Design review of the part built by this model. Coordinates are the model's own, in mm. A direction names the side the tool comes from. Coordinates: 2 decimals unless noted, no trailing zeros. Loops run counter-clockwise (first coordinate to the right, second up) from the corner with the lowest first, then second, coordinate; pieces in that order, holes last. Notation, with made-up numbers: (-7, 41.25) -> (8, 41.25) arc R5 cw to (8, 49.25) -> close; hole circle Ø9 at (73, 1). An arc over 180 degrees is marked (long way). One line per item, written item: value. Start each with the question number.
1. For probe 1 along Y at (x, z) = (9.5, 1); probe 2 along Y at (x, z) = (8, 16); probe 3 along Y at (x, z) = (9.75, 11), list the stretches that pass through material, from the lowest coordinate up.
2. Add section A-A on y = 52. Write out the cut boundary in (x, z).
3. Insertion check: pin 1 (12 mm diameter, centred on x = -2.5, z = 3.5, fed in from -Y); pin 2 (2.5 mm diameter, centred on x = 11.5, y = 99, fed in from -Z); pin 3 (4 mm diameter, centred on y = 100, z = 16, fed in from -X); pin 4 (12 mm diameter, centred on x = -6.5, z = -4, fed in from -Y). Each pin has a flat end and moves straight along its axis. Give the tip position at first contact, or say it passes through.
4. Draft analysis for pull direction Z (two halves, no side actions). For faces 4 (the flat face through (0, 15, 9)), 5 (the flat face through (-10, 100, 19.5)), 6 (the flat face through (2, 17, -7)), 7 (the flat face through (12.407, 107.068, 9.333)), state which applies: pulls with the +Z half, pulls with the -Z half, needs draft (parallel to the pull), parting line crosses it, or undercut.
5. Machinability: for faces 1 (the flat face through (7.5, 100, 18)), 2 (the flat face through (8.2, 0, -1.2)), 3 (the flat face through (-9, 98, 16)), which of the approach directions +Z, -Z, +X, -X, +Y, -Y give a long, thin tool a straight path to every point of the face, cutting with its end or side? Answer none if there is none.
6. Add section B-B on z = 0.5. Give the number of separate pieces and of enclosed holes in the cut face, plus the area to 3 significant figures.
```python
from build123d import *

# Parameters (mm, degrees)
BOSS_EXTRUDE1_DEPTH = 200
SKETCH4_R           = 7
CUT_EXTRUDE2_DEPTH  = 200
SKETCH3_W           = 20
SKETCH3_H           = 169
SKETCH3_W_2         = 21
SKETCH3_H_2         = 15
CUT_EXTRUDE1_DEPTH  = 100
SKETCH5_R           = 7.565
CUT_EXTRUDE3_DEPTH  = 6
CUT_EXTRUDE4_START  = -6
SKETCH6_R           = 7.565
CUT_EXTRUDE4_DEPTH  = 6
CUT_EXTRUDE8_START  = -100
SKETCH11_W          = 7
SKETCH11_H          = 2
CUT_EXTRUDE8_DEPTH  = 4
SKETCH13_W          = 16
SKETCH13_H          = 16
BOSS_EXTRUDE3_DEPTH = 4
SKETCH14_W          = 5
SKETCH14_H          = 15
CUT_EXTRUDE11_DEPTH = 203.546291005
CHAMFER1_SIZE       = 2
SKETCH15_W          = 23
SKETCH15_H          = 23
CUT_EXTRUDE12_DEPTH = 2
CUT_EXTRUDE13_DEPTH = 8
SKETCH17_R          = 1.55
CUT_EXTRUDE14_DEPTH = 203.546291005
SKETCH18_R          = 2.75
CUT_EXTRUDE15_DEPTH = 3.5
CUT_EXTRUDE16_DEPTH = 3.5
FILLET2_R           = 1


with BuildPart() as part:
    # Sketch1 → Boss-Extrude1 (new body)
    with BuildSketch(Plane(origin=(0, 0, 0), x_dir=(1, 0, 0), z_dir=(0, 1, 0))):
        with BuildLine():
            Line((-12.5, -10), (-10.894701926, 1.518377407))
            ThreePointArc((-10.894701926, 1.518377407), (0, 11), (10.894701926, 1.518377407))
            Line((10.894701926, 1.518377407), (12.5, -10))
            Line((12.5, -10), (12.5, -20))
            Line((12.5, -20), (-12.5, -20))
            Line((-12.5, -20), (-12.5, -10))
        make_face()
    extrude(amount=BOSS_EXTRUDE1_DEPTH)

    # Sketch4 → Cut-Extrude2 (cut)
    with BuildSketch(Plane.XZ):
        with Locations(Location((0, 0, 0), (0, 0, 270))):
            Circle(SKETCH4_R)
    extrude(amount=-CUT_EXTRUDE2_DEPTH, mode=Mode.SUBTRACT)

    # Sketch3 → Cut-Extrude1 (cut, symmetric)
    with BuildSketch(Plane(origin=(0, 0, 0), x_dir=(0, 0, -1), z_dir=(1, 0, 0))):
        with Locations((1, 107.5)):
            Rectangle(SKETCH3_W, SKETCH3_H)
        with Locations((0.5, 7.5)):
            Rectangle(SKETCH3_W_2, SKETCH3_H_2)
    extrude(amount=CUT_EXTRUDE1_DEPTH, both=True, mode=Mode.SUBTRACT)

    # Sketch5 → Cut-Extrude3 (cut)
    with BuildSketch(Plane.XZ.offset(-192)):
        with Locations(Location((0, 0, 0), (0, 0, 270))):
            Circle(SKETCH5_R)
    extrude(amount=-CUT_EXTRUDE3_DEPTH, mode=Mode.SUBTRACT)

    # Sketch6 → Cut-Extrude4 (cut)
    with BuildSketch(Plane(origin=(0, 23, 0), x_dir=(1, 0, 0), z_dir=(0, 1, 0)).offset(CUT_EXTRUDE4_START)):
        with Locations(Location((0, 0, 0), (0, 0, 90))):
            Circle(SKETCH6_R)
    extrude(amount=CUT_EXTRUDE4_DEPTH, mode=Mode.SUBTRACT)

    # Sketch11 → Cut-Extrude8 (cut, symmetric)
    with BuildSketch(Plane.XZ.offset(CUT_EXTRUDE8_START)):
        with Locations((-9, 20.5)):
            Rectangle(SKETCH11_W, SKETCH11_H)
    extrude(amount=CUT_EXTRUDE8_DEPTH, both=True, mode=Mode.SUBTRACT)

    # Sketch13 → Boss-Extrude3 (add)
    with BuildSketch(Plane.XZ):
        Polygon((-12.5, 20), (12.5, 20), (12.5, -12), (9.5, -15), (-9.5, -15), (-12.5, -12), align=None)
        Rectangle(SKETCH13_W, SKETCH13_H, mode=Mode.SUBTRACT)
    extrude(amount=BOSS_EXTRUDE3_DEPTH)

    # Sketch14 → Cut-Extrude11 (cut, through all)
    with BuildSketch(Plane.ZY.offset(12.5)):
        with Locations((12.5, 7.5)):
            Rectangle(SKETCH14_W, SKETCH14_H)
    extrude(amount=-CUT_EXTRUDE11_DEPTH, mode=Mode.SUBTRACT)

    # Chamfer1
    chamfer1_edges = [part.edges().sort_by_distance(p)[0] for p in [
        (0, 15, 15),
        (0, 0, 15),
    ]]
    chamfer(chamfer1_edges, length=CHAMFER1_SIZE)

    # Sketch15 → Cut-Extrude12 (cut)
    with BuildSketch(Plane.XZ.offset(4)):
        Rectangle(SKETCH15_W, SKETCH15_H)
    extrude(amount=-CUT_EXTRUDE12_DEPTH, mode=Mode.SUBTRACT)

    # Sketch16 → Cut-Extrude13 (cut)
    with BuildSketch(Plane.XY.offset(20)):
        Polygon((0, 108.660254038), (-7.5, 104.330127019), (-7.5, 95.669872981), (0, 91.339745962), (7.5, 95.669872981), (7.5, 104.330127019), align=None)
    extrude(amount=-CUT_EXTRUDE13_DEPTH, mode=Mode.SUBTRACT)

    # Sketch17 → Cut-Extrude14 (cut, through all)
    with BuildSketch(Plane.ZY.offset(12.5)):
        with Locations((16, 100)):
            Circle(SKETCH17_R)
    extrude(amount=-CUT_EXTRUDE14_DEPTH, mode=Mode.SUBTRACT)

    # Sketch18 → Cut-Extrude15 (cut)
    with BuildSketch(Plane.ZY.offset(12.5)):
        with Locations((16, 100)):
            Circle(SKETCH18_R)
    extrude(amount=-CUT_EXTRUDE15_DEPTH, mode=Mode.SUBTRACT)

    # Sketch19 → Cut-Extrude16 (cut)
    with BuildSketch(Plane(origin=(12.5, 0, 0), x_dir=(0, 0, -1), z_dir=(1, 0, 0))):
        Polygon((-16, 103.233161507), (-18.8, 101.616580754), (-18.8, 98.383419246), (-16, 96.766838493), (-13.2, 98.383419246), (-13.2, 101.616580754), align=None)
    extrude(amount=-CUT_EXTRUDE16_DEPTH, mode=Mode.SUBTRACT)

    # Fillet2
    # the kernel refuses this fillet: 1 mm, written as the material it takes off along each edge
    with BuildSketch(Plane(origin=(-12.5, 100, 16), x_dir=(0, 0, 1), z_dir=(0, -1, 0))) as fillet2_piece_1:
        with BuildLine():
            CenterArc((2.75 + FILLET2_R, -FILLET2_R), FILLET2_R, 90, 90)
            Line((2.75, -FILLET2_R), (2.75, 0))
            Line((2.75, 0), (2.75 + FILLET2_R, 0))
        make_face()
    revolve(axis=Axis((-12.5, 100, 16), (-1, 0, 0)), mode=Mode.SUBTRACT)


solid = part.part
```
Worked answers:
1. probe 1: y = -2 to 0, 15 to 23, 192 to 200
1. probe 2: y = -4 to 98.45, 101.55 to 200
1. probe 3: y = -2 to 0, 15 to 200
2. outline: (-12.5, 10) -> (-12.36, 9) -> (12.36, 9) -> (12.5, 10) -> (12.5, 20) -> (-12.5, 20) -> close
3. pin 1: stops at y = -2
3. pin 2: stops at z = 9
3. pin 3: stops at x = -9
3. pin 4: stops at y = -4
4. face 4: needs draft
4. face 5: pulls with the +Z half
4. face 6: undercut
4. face 7: pulls with the -Z half
5. face 1: +Z
5. face 2: -Z, +X, -X
5. face 3: -X
6. separate pieces: 6
6. enclosed holes: 0
6. area: 143 mm²
